The listing builds one solid part. Answer for the finished solid, in the listing's coordinates (mm). Face numbers are marked on the shaded views. Give positions to 0.01 mm unless a question says otherwise; leave off trailing zeros. Write each loop counter-clockwise with the first axis right and the second up, starting at its lowest first coordinate (ties: lowest second). Pieces come first, ordered by that corner, then holes. Notation, with made-up numbers: (35.25, 25.5) - (66.25, 25.5) arc R34 ccw to (66.25, 57.5) - close; hole circle Ø11 at (84, -6.5). An arc over 180 degrees is marked (long way). One line per item, written item: value. Start each with the question number.
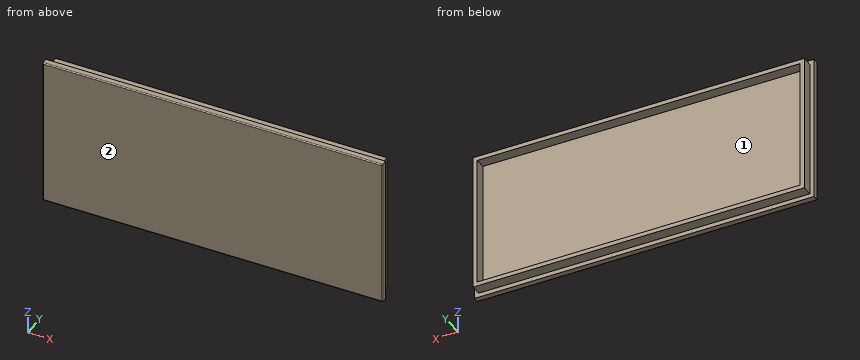
from build123d import *

# Parameters (mm, degrees)
SKETCH_1_W           = 160
SKETCH_1_H           = 70
SKETCH_1_W_2         = 156
SKETCH_1_H_2         = 66
EXTRUDE_1_DEPTH      = 3
EXTRUDE_2_DEPTH      = 5
EXTRUDE_2_DEPTH_BACK = 3
SKETCH_2_W           = 156
SKETCH_2_H           = 66
SKETCH_3_W           = 152
SKETCH_3_H           = 62
CUT_EXTRUDE_1_DEPTH  = 5
FILLET_1_R           = 0.5


with BuildPart() as part:
    # 스케치1 → 보스-돌출1 (new body)
    with BuildSketch(Plane(origin=(0, 0, 0), x_dir=(1, 0, 0), z_dir=(0, 1, 0))):
        Rectangle(SKETCH_1_W, SKETCH_1_H)
        Rectangle(SKETCH_1_W_2, SKETCH_1_H_2, mode=Mode.SUBTRACT)
    extrude(amount=EXTRUDE_1_DEPTH)

    # 스케치2 → 보스-돌출2 (add, two sides: drawn at the far end of the back side and taken through both)
    with BuildSketch(Plane(origin=(0, 3, 0), x_dir=(1, 0, 0), z_dir=(0, 1, 0)).offset(-EXTRUDE_2_DEPTH_BACK)):
        Rectangle(SKETCH_2_W, SKETCH_2_H)
    extrude(amount=EXTRUDE_2_DEPTH + EXTRUDE_2_DEPTH_BACK)

    # 스케치3 → 컷-돌출1 (cut)
    with BuildSketch(Plane(origin=(0, 8, 0), x_dir=(1, 0, 0), z_dir=(0, 1, 0))):
        Rectangle(SKETCH_3_W, SKETCH_3_H)
    extrude(amount=-CUT_EXTRUDE_1_DEPTH, mode=Mode.SUBTRACT)

    # 필렛1
    fillet_1_edges = [part.edges().sort_by_distance(p)[0] for p in [
        (0, 0, -35),
        (80, 0, 0),
        (0, 0, 35),
        (-80, 0, 0),
    ]]
    fillet(fillet_1_edges, radius=FILLET_1_R)


solid = part.part
Item 1: Straight lines are drawn through the part: line 1 along X through (y, z) = (5, 28); line 2 along Z through (x, y) = (-33, 3.5); line 3 along Y through (x, z) = (-53, -21). For each, find the intervals that lie inside material, in ascending order.
Item 2: Find section A-A on x = 2. Determine the outline of the cut face in (y, z).
Item 3: Each of these flat-tipped pins is pushed along its axis until it touches: pin 1 Ø2.5 at (y, z) = (6.5, -3.5) entering from +X; pin 2 Ø2.5 at (x, y) = (-13.5, 5.5) entering from -Z; pin 3 Ø6 at (x, z) = (-6, -3) entering from +Y. Where does it stop, or does it pass through?
Item 4: The mould has two halves that part along X. Classify the marked faces 1 and 2: +X half, -X half, draft (parallel to the pull), parting line (faces both ways), or undercut.
Item 5: Find section C-C on z = -26.5. Determine the outline of the cut face in (x, y).
Item 6: Find section B-B on y = 5.25. Determine the outline of the cut face in (x, z), plus the area to 3 significant figures.
Values:
1. line 1: -78 to -76, 76 to 78
1. line 2: -33 to -31, 31 to 33
1. line 3: 0 to 3
2. outline: (0, -34.5) arc R0.5 ccw to (0.5, -35) - (3, -35) - (3, -33) - (8, -33) - (8, -31) - (3, -31) - (3, 31) - (8, 31) - (8, 33) - (3, 33) - (3, 35) - (0.5, 35) arc R0.5 ccw to (0, 34.5) - close
3. pin 1: x = 78
3. pin 2: z = -33
3. pin 3: y = 3
4. face 1: undercut
4. face 2: draft
5. outline: (-80, 0.5) arc R0.5 ccw to (-79.5, 0) - (79.5, 0) arc R0.5 ccw to (80, 0.5) - (80, 3) - (78, 3) - (78, 8) - (76, 8) - (76, 3) - (-76, 3) - (-76, 8) - (-78, 8) - (-78, 3) - (-80, 3) - close
6. outline: (-78, -33) - (78, -33) - (78, 33) - (-78, 33) - close; hole (-76, -31) - (76, -31) - (76, 31) - (-76, 31) - close
6. area: 872 mm^2
